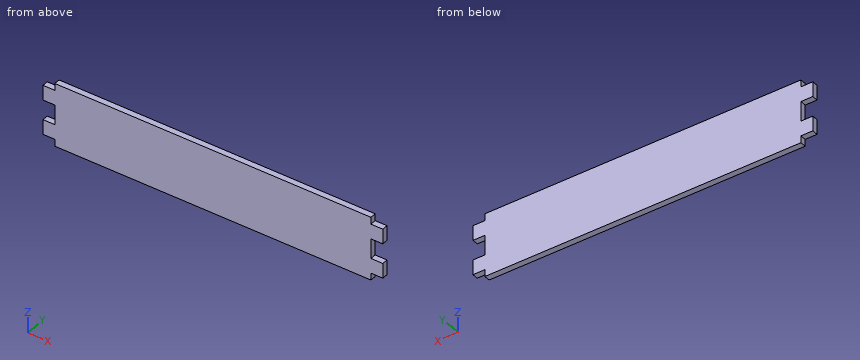
```python
from build123d import *

# Parameters (mm, degrees)
SKIZZE1_W                       = 320
SKIZZE1_H                       = 64
GRUNDFORM_DEPTH                 = 6
SKIZZE3_W                       = 15
SKIZZE3_H                       = 6
AUFSATZ_LINEAR_AUSTRAGEN2_DEPTH = 12


with BuildPart() as part:
    # Skizze1 → Grundform (new body)
    with BuildSketch(Plane(origin=(0, 0, 0), x_dir=(1, 0, 0), z_dir=(0, 1, 0))):
        Rectangle(SKIZZE1_W, SKIZZE1_H)
    extrude(amount=GRUNDFORM_DEPTH)

    # Skizze3 → Aufsatz-Linear austragen2 (add)
    with BuildSketch(Plane.ZY.offset(160)):
        with Locations((-17.5, 3)):
            Rectangle(SKIZZE3_W, SKIZZE3_H)
        with Locations((17.5, 3)):
            Rectangle(SKIZZE3_W, SKIZZE3_H)
    aufsatz_linear_austragen2 = extrude(amount=AUFSATZ_LINEAR_AUSTRAGEN2_DEPTH)

    # Spiegeln1: Aufsatz-Linear austragen2 across plane
    add(aufsatz_linear_austragen2.mirror(Plane(origin=(0, 0, 0), x_dir=(0, 0, 1), z_dir=(1, 0, 0))))


solid = part.part
```
The listing builds one solid part. Answer for the finished solid, in the listing's coordinates (mm). Round coordinates to 2 decimals unless told otherwise and drop trailing zeros. Loops run counter-clockwise (first coordinate to the right, second up) from the corner with the lowest first, then second, coordinate; pieces in that order, holes last.
1) Consider line 1 (X direction, y = 3.7, z = -26). Determine where the line is inside the solid, lowest interval first.
Outcome:
line 1: x = -160 to 160
2) Given P1, Ø1.8, axis at y = 4.5, z = -0.5, coming from the +X side; P2, Ø3, axis at x = -165.5, y = 4, coming from the -Z side; P3, Ø1.8, axis at x = 168.5, y = 4, coming from the +Z side, each flat-ended and moving along its own axis, determine where each tip first touches the part or whether it passes through.
Outcome:
P1: stops at x = 160
P2: stops at z = -25
P3: stops at z = 25
3) A cutting plane is placed at B-B on z = -3.5. Determine the outline of the cut face in (x, y).
Outcome:
outline: (-160, 0) - (160, 0) - (160, 6) - (-160, 6) - close
4) A cutting plane is placed at A-A on y = 3.8. Determine the outline of the cut face in (x, z), plus the area to 3 significant figures.
Outcome:
outline: (-172, -25) - (-160, -25) - (-160, -32) - (160, -32) - (160, -25) - (172, -25) - (172, -10) - (160, -10) - (160, 10) - (172, 10) - (172, 25) - (160, 25) - (160, 32) - (-160, 32) - (-160, 25) - (-172, 25) - (-172, 10) - (-160, 10) - (-160, -10) - (-172, -10) - close
area: 21,200 mm2
